from build123d import *

# Parameters (mm, degrees)
F0_R     = 11
F1_DEPTH = 14
F2_R     = 4
F3_DEPTH = 10
F4_R     = 11.274744
F4_R_2   = 6.443865
F5_DEPTH = 6


with BuildPart() as f1:
    # F0 (on Front) → F1 (new body)
    with BuildSketch(Plane.XZ):
        with BuildLine():
            Line((7.46888, 13.008299), (0, 15))
            ThreePointArc((0, 15), (-15, 0), (0, -15))
            Line((0, -15), (7.46888, -13.008299))
            ThreePointArc((7.46888, -13.008299), (12.981394, -7.515544), (15, 0))
            ThreePointArc((15, 0), (12.981394, 7.515544), (7.46888, 13.008299))
        make_face()
        Circle(F0_R, mode=Mode.SUBTRACT)
        with BuildLine():
            ThreePointArc((7.46888, 13.008299), (3.86494, 14.493524), (0, 15))
            Line((0, 15), (7.46888, 13.008299))
        make_face()
        with BuildLine():
            Line((7.46888, -13.008299), (0, -15))
            ThreePointArc((0, -15), (3.86494, -14.493524), (7.46888, -13.008299))
        make_face()
        with BuildLine():
            Line((30, 7), (7.46888, 13.008299))
            ThreePointArc((7.46888, 13.008299), (12.981394, 7.515544), (15, 0))
            ThreePointArc((15, 0), (12.981394, -7.515544), (7.46888, -13.008299))
            Line((7.46888, -13.008299), (30, -7))
            Line((30, -7), (30, 0))
            Line((30, 0), (30, 7))
        make_face()
    extrude(amount=F1_DEPTH)

    # F2 (on face) → F3 (cut)
    with BuildSketch(Plane.YZ.offset(30)):
        with Locations((-7, 0)):
            Circle(F2_R)
    extrude(amount=-F3_DEPTH, mode=Mode.SUBTRACT)

    # F4 (on face) → F5 (join)
    with BuildSketch(Plane.XZ.offset(14)):
        Circle(F4_R)
        Circle(F4_R_2, mode=Mode.SUBTRACT)
    extrude(amount=-F5_DEPTH)


solid = f1.part
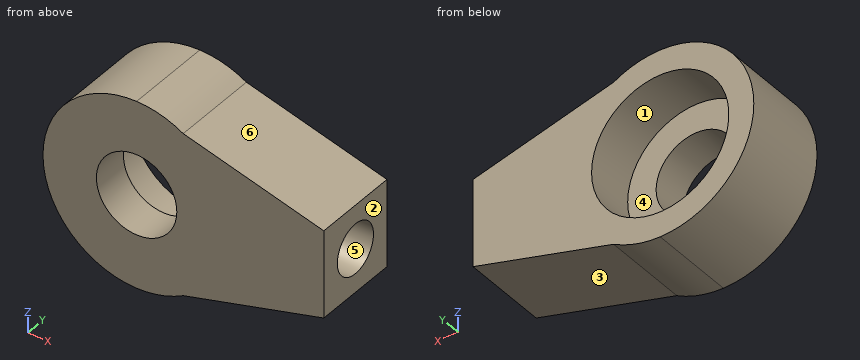
Geometry check sheet. Reference: the model listing, model coordinates, mm. Face numbers are marked on the shaded views. A direction names the side the tool comes from. Round coordinates to 2 decimals unless told otherwise and drop trailing zeros. Write each loop counter-clockwise with the first axis right and the second up, starting at its lowest first coordinate (ties: lowest second). Pieces come first, ordered by that corner, then holes. Notation, with made-up numbers: (40.5, 87.25) - (50.5, 87.25) arc R16 cw to (50.5, 101.25) - close; hole circle Ø2 at (58.25, 33.5). An arc over 180 degrees is marked (long way). One line per item, written item: value.
1. Set-up check for the marked faces 5 and 6: record each of +Z, -Z, +X, -X, +Y, -Y from which the full face is reachable in a straight line by a thin tool's end or side.
The answers:
face 5: +X
face 6: +Z, +X, +Y, -Y
2. Cross-section at D-D on y = -2.25. Record the boundary of the cut face in (x, z), and give its area (3 significant figures).
The answers:
outline: (0, -15) arc R15 ccw to (7.47, -13.01) - (30, -7) - (30, 7) - (7.47, 13.01) arc R15 ccw to (0, 15) arc R15 ccw to start; hole circle Ø22 at (0, 0)
area: 639 mm^2
3. Scan lines: L1, parallel to X at y = -10.5, z = 0.25; L2, parallel to X at y = -2, z = 0; L3, parallel to Y at x = 6, z = 5.75. Record each from-to range of solid material in increasing order.
The answers:
L1: x = -15 to -6.44, 6.44 to 20
L2: x = -15 to -11, 11 to 30
L3: y = -14 to -8
4. Cross-section at C-C on x = 0.5. Record the boundary of the cut face in (y, z), and give its area (3 significant figures).
The answers:
outline: (-14, -14.99) - (0, -14.99) - (0, -10.99) - (-8, -10.99) - (-8, -6.42) - (-14, -6.42) - close; (-14, 6.42) - (-8, 6.42) - (-8, 10.99) - (0, 10.99) - (0, 14.99) - (-14, 14.99) - close
area: 167 mm^2
5. Cross-section at A-A on y = -12.25. Record the boundary of the cut face in (x, z), and give its area (3 significant figures).
The answers:
outline: (0, -15) arc R15 ccw to (7.47, -13.01) - (30, -7) - (30, 7) - (7.47, 13.01) arc R15 ccw to (0, 15) arc R15 ccw to start; hole circle Ø12.89 at (0, 0)
area: 888 mm^2
6. Depth check by flat-ended pin: pin 1 Ø2 at (x, y) = (-4.5, -5.5) entering from -Z; pin 2 Ø1 at (y, z) = (-4.5, 7.5) entering from -X; pin 3 Ø10.5 at (x, z) = (0, 0) entering from -Y; pin 4 Ø6.5 at (y, z) = (-7, -0.5) entering from +X. Enter the tip coordinate at first touch or a pass-through.
The answers:
pin 1: stops at z = -14.59
pin 2: stops at x = -13.27
pin 3: passes through
pin 4: stops at x = 20
7. Cross-section at B-B on z = 0. Record the boundary of the cut face in (x, y), and give its area (3 significant figures).
The answers:
outline: (-15, -14) - (-6.44, -14) - (-6.44, -8) - (-11, -8) - (-11, 0) - (-15, 0) - close; (6.44, -14) - (30, -14) - (30, -11) - (20, -11) - (20, -3) - (30, -3) - (30, 0) - (11, 0) - (11, -8) - (6.44, -8) - close
area: 297 mm^2
8. Mould release check, pull along Z, two halves, no side actions. Record for the marked faces 1, 2, 3 and 4: released by +Z, released by -Z, zero draft, split by the parting line, or undercut.
The answers:
face 1: undercut
face 2: zero draft
face 3: released by -Z
face 4: undercut
